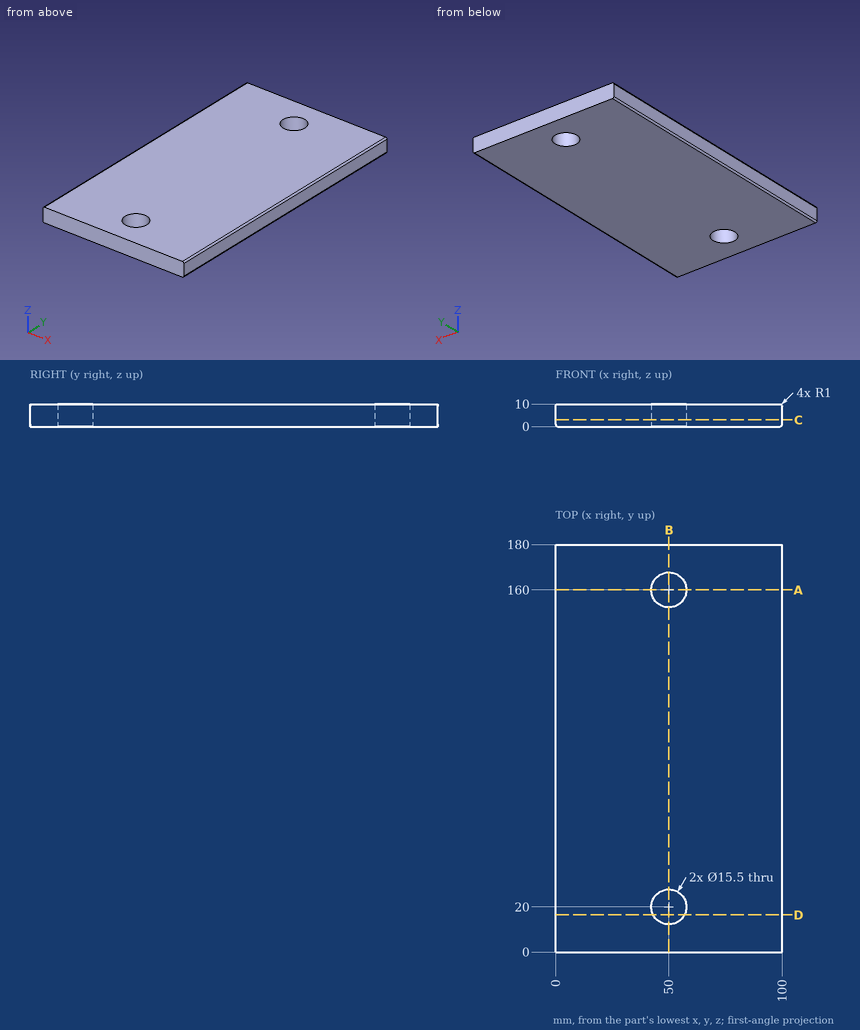
For this review, use the dimensioned drawing (mm, ordinates from the lowest corner) and the shaded views. Coordinates: 2 decimals unless noted, no trailing zeros. Write each loop counter-clockwise with the first axis right and the second up, starting at its lowest first coordinate (ties: lowest second). Pieces come first, ordered by that corner, then holes. Notation, with made-up numbers: (-25.5, 4) - (16.5, 4) arc R24 ccw to (16.5, 26) - close; hole circle Ø6 at (7, 72). An arc over 180 degrees is marked (long way). Answer in a Markdown table with one row per item. Add a question column.
Q1. Consider section D-D on y = 16.5. Give the boundary of the cut face in (x, z), then the cut area to 3 significant figures.
Q2. To check wall thickness, follow line 1 along Y through (x, z) = (50, 5.5); line 2 along Y through (x, z) = (55.5, 9.5); line 3 along X through (y, z) = (14, 1). State the ranges of each line that lie inside material, in increasing order. Write a range as from..to.
Q3. Consider section B-B on x = 50. Give the boundary of the cut face in (y, z), then the cut area to 3 significant figures.
Q4. Consider section A-A on y = 160. Give the boundary of the cut face in (x, z).
Q5. Consider section C-C on z = 3. Give the boundary of the cut face in (x, y), then the cut area to 3 significant figures.
Answers below:
| question | item | result |
|---|---|---|
| 1 | outline | (0, 1) arc R1 ccw to (1, 0) - (43.09, 0) - (43.09, 10) - (1, 10) arc R1 ccw to (0, 9) - close; (56.91, 0) - (99, 0) arc R1 ccw to (100, 1) - (100, 9) arc R1 ccw to (99, 10) - (56.91, 10) - close |
| 1 | area | 861 mm² |
| 2 | line 1 | 0..12.25, 27.75..152.25, 167.75..180 |
| 2 | line 2 | 0..14.54, 25.46..154.54, 165.46..180 |
| 2 | line 3 | 0..45.09, 54.91..100 |
| 3 | outline | (0, 0) - (12.25, 0) - (12.25, 10) - (0, 10) - close; (27.75, 0) - (152.25, 0) - (152.25, 10) - (27.75, 10) - close; (167.75, 0) - (180, 0) - (180, 10) - (167.75, 10) - close |
| 3 | area | 1,490 mm² |
| 4 | outline | (0, 1) arc R1 ccw to (1, 0) - (42.25, 0) - (42.25, 10) - (1, 10) arc R1 ccw to (0, 9) - close; (57.75, 0) - (99, 0) arc R1 ccw to (100, 1) - (100, 9) arc R1 ccw to (99, 10) - (57.75, 10) - close |
| 5 | outline | (0, 0) - (100, 0) - (100, 180) - (0, 180) - close; hole circle Ø15.5 at (50, 20); hole circle Ø15.5 at (50, 160) |
| 5 | area | 17,600 mm² |
